```python
from build123d import *

# Parameters (mm, degrees)
F0_R     = 110
F1_DEPTH = 12.5
F3_DEPTH = 25
F4_R     = 67.5
F5_DEPTH = 21
F6_R     = 40
F7_DEPTH = 60


with BuildPart() as f1:
    # F0 (on Top) → F1 (new body, symmetric)
    with BuildSketch(Plane.XY):
        Circle(F0_R)
    extrude(amount=F1_DEPTH, both=True)

    # F2 (on face) → F3 (join)
    with BuildSketch(Plane.XY.offset(12.5)):
        Polygon((-110, 0), (110, 0), (150, 410), (-150, 410), align=None)
    extrude(amount=-F3_DEPTH)

    # F4 (on face) → F5 (join)
    with BuildSketch(Plane(origin=(0, 0, -12.5), x_dir=(1, 0, 0), z_dir=(0, 0, -1))):
        Circle(F4_R)
    extrude(amount=F5_DEPTH)

    # F6 (on face) → F7 (cut)
    with BuildSketch(Plane(origin=(0, 0, -33.5), x_dir=(1, 0, 0), z_dir=(0, 0, -1))):
        Circle(F6_R)
    extrude(amount=-F7_DEPTH, mode=Mode.SUBTRACT)


solid = f1.part
```
The model under review builds one solid part; all positions refer to its coordinate system, in mm. A direction names the side the tool comes from. Coordinates: 2 decimals unless noted, no trailing zeros. Order: outer loops, then holes, each group sorted by start corner. A loop starts at its lowest first (then second) coordinate and runs counter-clockwise, first axis right, second up. Notation, with made-up numbers: M 75,-23 L 101,-23 A22 cw 101,11 Z; hole C 41.5,25.25 d3. An arc over 180 degrees is marked long. One line per question, with ' | ' between items.
(1) Add section B-B, the plane z = -4. Write out the cut boundary in (x, y), then the cut area to 3 significant figures.
Geometry results:
outline: M -150,410 L -110,0 A110 ccw 110,0 L 150,410 Z; hole C 0,0 d80 | area: 121,000 mm²
(2) Add section C-C, the plane y = 129. Write out the cut boundary in (x, z).
Geometry results:
outline: M -122.59,-12.5 L 122.59,-12.5 L 122.59,12.5 L -122.59,12.5 Z
(3) Add section A-A, the plane x = 0. Write out the cut boundary in (y, z).
Geometry results:
outline: M -110,-12.5 L -67.5,-12.5 L -67.5,-33.5 L -40,-33.5 L -40,12.5 L -110,12.5 Z; M 40,-33.5 L 67.5,-33.5 L 67.5,-12.5 L 410,-12.5 L 410,12.5 L 40,12.5 Z
(4) Machinability: for faces 4 (the face through (-53.57, 41.07, -22.85)), 5 (the face through (2, 410, 0)), which of the approach directions +Z, -Z, +X, -X, +Y, -Y give a long, thin tool a straight path to every point of the face, cutting with its end or side? Answer none if there is none.
Geometry results:
face 4: -Z | face 5: +Z, -Z, +X, -X, +Y
(5) The part is to be moulded in two halves that separate along Y. For faces 1 (the face through (-2, 211, 12.5)), 2 (the face through (-8.67, 39.05, -10.82)), 3 (the face through (-2.419, -109.973, 0.175)), say which applies: +Y half, -Y half, draft (parallel to the pull), parting line (faces both ways), or undercut.
Geometry results:
face 1: draft | face 2: undercut | face 3: -Y half
(6) Insertion check: pin 1 (5 mm diameter, centred on x = -41.5, z = 7.5, fed in from -Y); pin 2 (6 mm diameter, centred on x = 87.5, y = 145, fed in from -Z); pin 3 (4 mm diameter, centred on y = 43.5, z = -2, fed in from +X). Each pin has a flat end and moves straight along its axis. Give the tip position at first contact, or say it passes through.
Geometry results:
pin 1: stops at y = -102.85 | pin 2: stops at z = -12.5 | pin 3: stops at x = 114.44
(7) Add section D-D, the plane z = -28.5. Write out the cut boundary in (x, y).
Geometry results:
outline: C 0,0 d135; hole C 0,0 d80
(8) For probe 1 along X at (y, z) = (0, -17.5); probe 2 along Y at (x, z) = (0, -9), list the stretches that pass through material, from the lowest coordinate up. Write a range as from..to.
Geometry results:
probe 1: x = -67.5..-40, 40..67.5 | probe 2: y = -110..-40, 40..410
